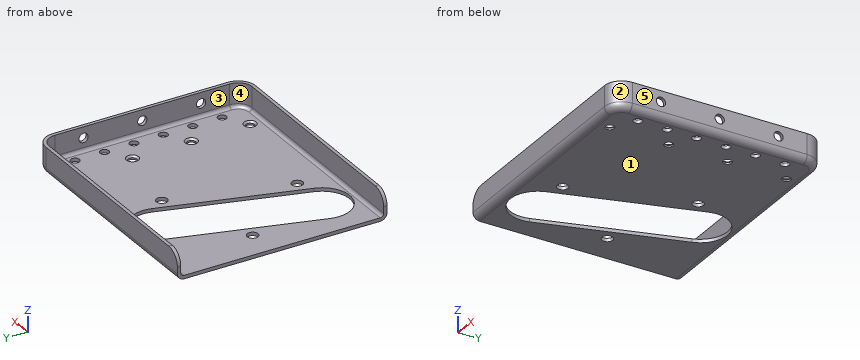
from build123d import *

# Parameters (mm, degrees)
F0_W            = 86.4
F0_H            = 77
F1_DEPTH        = 10
F2_R            = 6.4
F3_R            = 5.1
F4_R            = 2.5
F5_T            = -1.25
F7_DEPTH        = 1.251
F9_D            = 4
F11_D           = 3.2
F13_D           = 3.4
F15_D           = 3.2
F15_CSINK_D     = 4.5
F15_CSINK_ANGLE = 90


with BuildPart() as f1:
    # F0 (on Top) → F1 (new body)
    with BuildSketch(Plane.XY):
        with Locations((-43.2, 0)):
            Rectangle(F0_W, F0_H)
    extrude(amount=F1_DEPTH)

    # F2
    f2_edges = [f1.edges().sort_by_distance(p)[0] for p in [
        (0, 38.5, 5),
        (0, -38.5, 5),
    ]]
    fillet(f2_edges, radius=F2_R)

    # F3
    f3_edges = [f1.edges().sort_by_distance(p)[0] for p in [
        (-86.4, 0, 10),
    ]]
    fillet(f3_edges, radius=F3_R)

    # F4
    f4_edges = [f1.edges().sort_by_distance(p)[0] for p in [
        (-46.4, -38.5, 0),
    ]]
    fillet(f4_edges, radius=F4_R)

    # F5
    f5_openings = [f1.faces().sort_by_distance(p)[0] for p in [
        (-86.4, 0, 2.463545),
        (-84.906245, 0, 8.506245),
        (-40.760453, 0, 10),
    ]]
    offset(amount=F5_T, openings=f5_openings)

    # F6 (on face) → F7 (cut, through all)
    with BuildSketch(Plane.XY.offset(1.25)):
        with BuildLine():
            ThreePointArc((-78.6069464832, -22.3663473264), (-71.8133409919, -34.9308578393), (-59.248830479, -28.1372523479))
            Line((-59.248830479, -28.1372523479), (-44.1930535168, 22.3663473264))
            ThreePointArc((-44.1930535168, 22.3663473264), (-50.9866590081, 34.9308578393), (-63.551169521, 28.1372523479))
            Line((-63.551169521, 28.1372523479), (-78.6069464832, -22.3663473264))
        make_face()
    extrude(amount=-F7_DEPTH, mode=Mode.SUBTRACT)

    # F9 (through all)
    with Locations(Plane.XY.offset(1.25)):
        with Locations((-75.2956773297, 4.1424813274), (-41.2191785873, 16.9406153109), (-53.7894667532, -25.2255779656)):
            Hole(F9_D / 2)

    # F11 (through all)
    with Locations(Plane.XY.offset(1.25)):
        with Locations((-5.1, -27), (-5.1, -16.2), (-5.1, -5.4), (-5.1, 5.4), (-5.1, 16.2), (-5.1, 27)):
            Hole(F11_D / 2)

    # F13 (through all)
    with Locations(Plane.YZ):
        with Locations((-21.6, 6), (0, 6), (21.6, 6)):
            Hole(F13_D / 2)

    # F15 (through all)
    with Locations(Plane.XY.offset(1.25)):
        with Locations((-13.2, -32.4), (-13.2, -10.8), (-13.2, 10.8), (-13.2, 32.4)):
            CounterSinkHole(F15_D / 2, F15_CSINK_D / 2, counter_sink_angle=F15_CSINK_ANGLE)


solid = f1.part
Read the model definition and answer for the solid it produces. Units are mm, in the model's axes. Face numbers are marked on the shaded views. A direction names the side the tool comes from. Round coordinates to 2 decimals unless told otherwise and drop trailing zeros. Write each loop counter-clockwise with the first axis right and the second up, starting at its lowest first coordinate (ties: lowest second). Pieces come first, ordered by that corner, then holes.
1. Straight lines are drawn through the part: L1, parallel to Y at x = -63.5, z = 9; L2, parallel to X at y = -11, z = 1; L3, parallel to X at y = 10.8, z = 0.4. For each, find the intervals that lie inside material, in ascending order.
2. The part is cut by section D-D, the plane y = 27. Determine the outline of the cut face in (x, z).
3. The part is cut by section B-B, the plane z = 6. Determine the outline of the cut face in (x, y), then the cut area to 3 significant figures.
4. The part is cut by section C-C, the plane x = -33. Determine the outline of the cut face in (y, z).
5. Determine the mould class of the marked faces 1, 2 and 3 for opening direction Y: pulls with the +Y half, pulls with the -Y half, needs draft (parallel to the pull), parting line crosses it, or undercut.
6. Given pin 1 Ø10 at (x, y) = (-28.5, -0.5) entering from +Z; pin 2 Ø5.5 at (y, z) = (21.6, 6) entering from +X; pin 3 Ø4 at (y, z) = (0, 6) entering from -X; pin 4 Ø3.5 at (x, y) = (-13.2, -10.8) entering from +Z, each flat-ended and moving along its own axis, determine where each tip first touches the part or whether it passes through.
7. The part is cut by section A-A, the plane y = -5.4. Determine the outline of the cut face in (x, z), then the cut area to 3 significant figures.
8. Which of the six approach directions +Z, -Z, +X, -X, +Y, -Y give full straight-line access (tool end or side, diameter ignored) to the marked faces 4 and 5?
Values:
1. L1: y = -38.5 to -37.25, 37.25 to 38.5
1. L2: x = -86.4 to -75.22, -54.14 to -15.19, -11.21 to -0.5
1. L3: x = -86.4 to -68.72, -47.64 to -14.8, -11.6 to -1.14
2. outline: (-86.4, 0) - (-63.89, 0) - (-63.89, 1.25) - (-86.4, 1.25) - close; (-43.92, 0) - (-6.7, 0) - (-6.7, 1.25) - (-43.92, 1.25) - close; (-3.5, 0) - (-2.5, 0) arc R2.5 ccw to (0, 2.5) - (0, 10) - (-1.25, 10) - (-1.25, 2.5) arc R1.25 cw to (-2.5, 1.25) - (-3.5, 1.25) - close
3. outline: (-86.28, -38.5) - (-6.4, -38.5) arc R6.4 ccw to (0, -32.1) - (0, -23.3) - (-1.25, -23.3) - (-1.25, -32.1) arc R5.15 cw to (-6.4, -37.25) - (-86.28, -37.25) - close; (-86.28, 37.25) - (-6.4, 37.25) arc R5.15 cw to (-1.25, 32.1) - (-1.25, 23.3) - (0, 23.3) - (0, 32.1) arc R6.4 ccw to (-6.4, 38.5) - (-86.28, 38.5) - close; (-1.25, -19.9) - (0, -19.9) - (0, -1.7) - (-1.25, -1.7) - close; (-1.25, 1.7) - (0, 1.7) - (0, 19.9) - (-1.25, 19.9) - close
3. area: 290 mm2
4. outline: (-38.5, 2.5) arc R2.5 ccw to (-36, 0) - (36, 0) arc R2.5 ccw to (38.5, 2.5) - (38.5, 10) - (37.25, 10) - (37.25, 2.5) arc R1.25 cw to (36, 1.25) - (-36, 1.25) arc R1.25 cw to (-37.25, 2.5) - (-37.25, 10) - (-38.5, 10) - close
5. face 1: needs draft
5. face 2: pulls with the -Y half
5. face 3: undercut
6. pin 1: stops at z = 1.25
6. pin 2: stops at x = 0
6. pin 3: stops at x = -1.25
6. pin 4: stops at z = 0.75
7. outline: (-86.4, 0) - (-73.55, 0) - (-73.55, 1.25) - (-86.4, 1.25) - close; (-52.47, 0) - (-6.7, 0) - (-6.7, 1.25) - (-52.47, 1.25) - close; (-3.5, 0) - (-2.5, 0) arc R2.5 ccw to (0, 2.5) - (0, 10) - (-1.25, 10) - (-1.25, 2.5) arc R1.25 cw to (-2.5, 1.25) - (-3.5, 1.25) - close
7. area: 87.6 mm2
8. face 4: +Z, -X
8. face 5: +Z, -Z, +X, +Y, -Y
